Check sheet for the drawn part. Datum: minimum x, y, z corner. Units: mm. A direction names the side the tool comes from. Coordinates: 2 decimals unless noted, no trailing zeros. Write each loop counter-clockwise with the first axis right and the second up, starting at its lowest first coordinate (ties: lowest second). Pieces come first, ordered by that corner, then holes. Notation, with made-up numbers: (34, -32.75) -> (42, -32.75) arc R18 cw to (42, -9.75) -> close; hole circle Ø4 at (88.5, -24.75). An arc over 180 degrees is marked (long way). One line per question, with ' | ' between items.
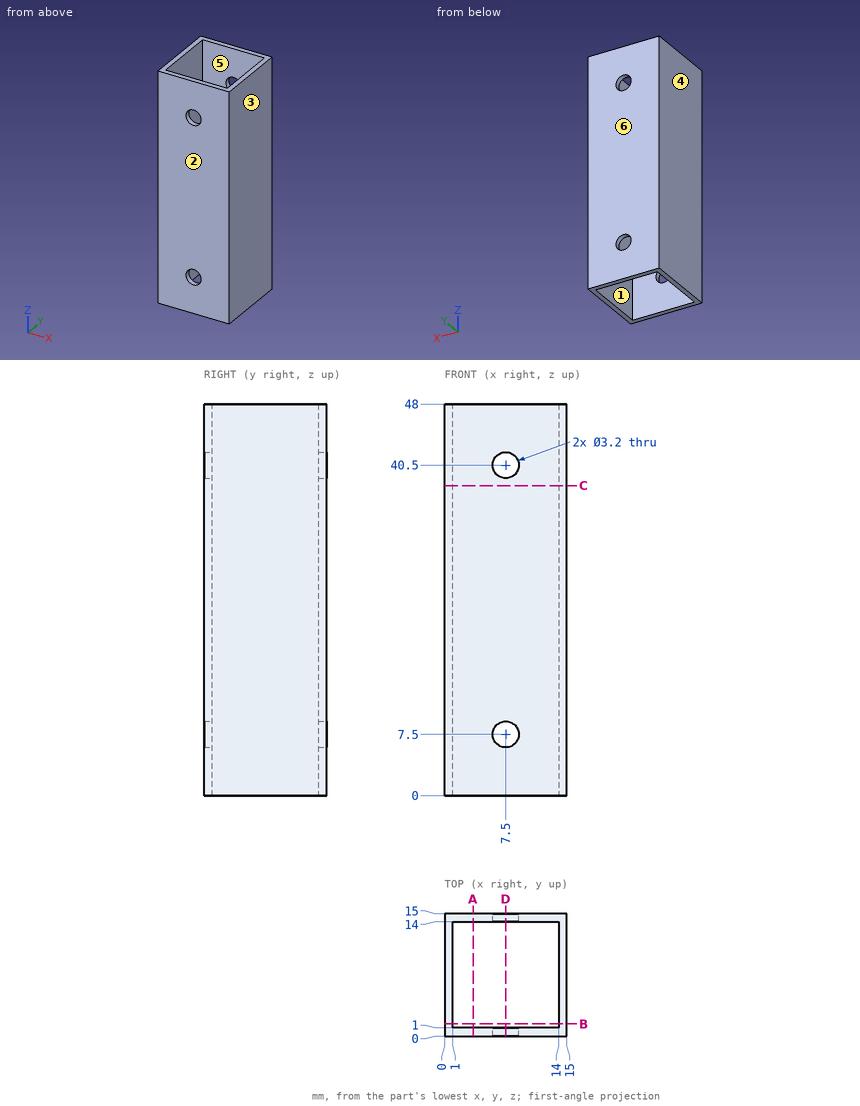
1. Tool access check on the marked faces 1 and 2. Record the directions out of +Z, -Z, +X, -X, +Y, -Y that give a thin tool (end or side, any length) a straight path to the whole face; none if there is none.
Worked answers:
face 1: +Z, -Z | face 2: +Z, -Z, +X, -X, -Y
2. Cross-section at D-D on x = 7.5. Record the boundary of the cut face in (y, z), and give its area (3 significant figures).
Worked answers:
outline: (0, 0) -> (1, 0) -> (1, 5.9) -> (0, 5.9) -> close; (0, 9.1) -> (1, 9.1) -> (1, 38.9) -> (0, 38.9) -> close; (0, 42.1) -> (1, 42.1) -> (1, 48) -> (0, 48) -> close; (14, 0) -> (15, 0) -> (15, 5.9) -> (14, 5.9) -> close; (14, 9.1) -> (15, 9.1) -> (15, 38.9) -> (14, 38.9) -> close; (14, 42.1) -> (15, 42.1) -> (15, 48) -> (14, 48) -> close | area: 83.2 mm²
3. Material ranges on line 1 (Z direction, x = 7.5, y = 14.6); line 2 (X direction, y = 0.45, z = 40.5); line 3 (Y direction, x = 5.25, z = 25), recorded low to high. Write a range as from..to.
Worked answers:
line 1: 0..5.9, 9.1..38.9, 42.1..48 | line 2: 0..5.9, 9.1..15 | line 3: 0..1, 14..15
4. Mould release check, pull along X, two halves, no side actions. Record for the marked faces 3, 4, 5 and 6: released by +X, released by -X, zero draft, split by the parting line, or undercut.
Worked answers:
face 3: released by +X | face 4: released by -X | face 5: undercut | face 6: zero draft
5. Cross-section at C-C on z = 38. Record the boundary of the cut face in (x, y).
Worked answers:
outline: (0, 0) -> (15, 0) -> (15, 15) -> (0, 15) -> close; hole (1, 1) -> (14, 1) -> (14, 14) -> (1, 14) -> close
6. Cross-section at A-A on x = 3.5. Record the boundary of the cut face in (y, z), and give its area (3 significant figures).
Worked answers:
outline: (0, 0) -> (1, 0) -> (1, 48) -> (0, 48) -> close; (14, 0) -> (15, 0) -> (15, 48) -> (14, 48) -> close | area: 96.0 mm²
